The listing builds one solid part. Answer for the finished solid, in the listing's coordinates (mm). Face numbers are marked on the shaded views. Coordinates: 2 decimals unless noted, no trailing zeros. Order: outer loops, then holes, each group sorted by start corner. A loop starts at its lowest first (then second) coordinate and runs counter-clockwise, first axis right, second up. Notation, with made-up numbers: (48, 56) -> (92, 56) arc R23 cw to (92, 81) -> close; hole circle Ø1 at (-14.5, 49.25). An arc over 180 degrees is marked (long way). Return JSON: item names as keys, results as strings.
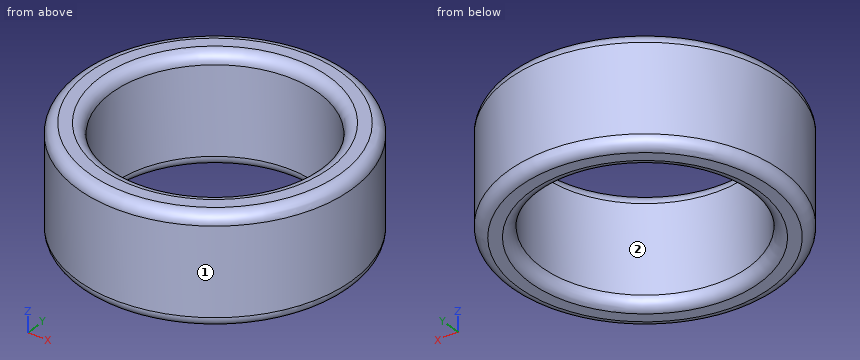
```python
from build123d import *

# Parameters (mm, degrees)
F0_R     = 31.964339
F1_DEPTH = 25.4
F2_R     = 24.135633
F3_DEPTH = 25.401
F4_R     = 2.54


with BuildPart() as f1:
    # F0 (on Top) → F1 (new body)
    with BuildSketch(Plane.XY):
        with Locations((-24.393266, 20.656416)):
            Circle(F0_R)
    extrude(amount=F1_DEPTH)

    # F2 (on face) → F3 (cut, through all)
    with BuildSketch(Plane.XY.offset(25.4)):
        with Locations((-24.393266, 20.656416)):
            Circle(F2_R)
    extrude(amount=-F3_DEPTH, mode=Mode.SUBTRACT)

    # F4
    f4_edges = [f1.edges().sort_by_distance(p)[0] for p in [
        (-56.357605, 20.656416, 25.4),
        (-56.357605, 20.656416, 0),
        (7.571073, 20.656416, 12.7),
        (-48.528899, 20.656416, 25.4),
        (-48.528899, 20.656416, 0),
    ]]
    fillet(f4_edges, radius=F4_R)


solid = f1.part
```
Item 1: Find the intervals of material crossed by probe 1 along Z at (x, y) = (2, 24); probe 2 along Y at (x, z) = (-27, 9); probe 3 along X at (y, z) = (40, 4.75), in increasing order.
Answer list:
{"probe 1": "0 to 25.4", "probe 2": "-11.2 to -3.34, 44.65 to 52.51", "probe 3": "-49.84 to -38.83, -9.96 to 1.05"}
Item 2: Determine the mould class of the marked faces 1 and 2 for opening direction Y: pulls with the +Y half, pulls with the -Y half, needs draft (parallel to the pull), parting line crosses it, or undercut.
Answer list:
{"face 1": "parting line crosses it", "face 2": "undercut"}
Item 3: Flat-ended cylindrical pins translate along their axes: pin 1 (8 mm diameter, centred on x = -17.5, z = 5, fed in from +Y); pin 2 (12 mm diameter, centred on y = 2, z = 8.5, fed in from -X); pin 3 (5 mm diameter, centred on x = -13.5, y = 3, fed in from +Z); pin 4 (5 mm diameter, centred on x = -1, z = 13.5, fed in from -Y). Find the tip coordinate at first contact, or state that the pin passes through.
Answer list:
{"pin 1": "y = 52.49", "pin 2": "x = -53.75", "pin 3": "through", "pin 4": "y = -3.53"}
Item 4: The part is cut by section A-A on z = 15.5. Determine the outline of the cut face in (x, y), plus the area to 3 significant figures.
Answer list:
{"outline": "circle Ø63.93 at (-24.39, 20.66); hole circle Ø48.27 at (-24.39, 20.66)", "area": "1,380 mm2"}
